The model under review builds one solid part; all positions refer to its coordinate system, in mm. Coordinates: 2 decimals unless noted, no trailing zeros. Write each loop counter-clockwise with the first axis right and the second up, starting at its lowest first coordinate (ties: lowest second). Pieces come first, ordered by that corner, then holes.
1) Mouldability with a two-part tool opening along Y and no side actions: class faces 1 (the cylindrical face through (1.57, 47.65, -37.69)), 2 (the flat face through (2, 51, 25.4)), 3 (the flat face through (1.57, 19.32, 12.88)) as released by +Y, released by -Y, zero draft, split by the parting line, or undercut.
2) Add section B-B, the plane z = -12.7. State the section outline as (x, y) points (3 decimals).
3) Add section A-A, the plane y = 50.8. State the section outline as (x, z) points (3 decimals), then the cut area to 3 significant figures.
4) For P1, Ø1, axis at x = 2, y = 28.5, coming from the +Z side, flat-tipped, find the tip position at first contact; note if it passes through.
5) Add section D-D, the plane y = 15. State the section outline as (x, z) points (3 decimals).
6) For line 1 (Z direction, x = 2.05, y = 50.8) (3 decimals); line 2 (Y direction, x = 1.2, z = -12.7) (3 decimals); line 3 (Z direction, x = 0.7, y = 48), list the stretches that pass through material, from the lowest coordinate up.
7) Add section C-C, the plane x = 2.1. State the section outline as (y, z) points (3 decimals).
Autodesk Inventor part; units mm, degrees
ref_plane "YZ Plane" through (0, 0, 0) normal (1, 0, 0) x (0, 1, 0)
ref_plane "XZ Plane" through (0, 0, 0) normal (0, 1, 0) x (-1, 0, 0)
ref_plane "XY Plane" through (0, 0, 0) normal (0, 0, 1) x (1, 0, 0)
sketch "Sketch1" plane through (0, 0, 0) normal (1, 0, 0) x (0, 1, 0)
  line L0 (0, 0) -> (0, -25.4)
  line L1 (0, -25.4) -> (38.1, -50.8)
  line L2 (38.1, -50.8) -> (63.5, -50.8)
  line L3 (63.5, -50.8) -> (63.5, 25.4)
  line L4 (63.5, 25.4) -> (38.1, 25.4)
  line L5 (38.1, 25.4) -> (0, 0)
  dimension "d0" = 76.2
  dimension "d2" = 25.4
  dimension "d3" = 25.4
  dimension "d4" = 25.4
  dimension "d5" = 63.5
  dimension "d6" = 25.4
extrude "Extrusion1" add sketch "Sketch1" along normal blind 3.175
sketch "Sketch2" plane through (3.175, 0, 0) normal (1, 0, 0) x (0, 0, -1)
  line L0 (0, 0) -> (25.4, 0)
  line L1 (50.8, 38.1) -> (50.8, 63.5)
  line L2 (50.8, 63.5) -> (-25.4, 63.5)
  line L3 (-25.4, 63.5) -> (-25.4, 38.1)
  point P0 (-12.7, 50.8)
  point P1 (38.1, 50.8)
  point P2 (12.7, 12.7)
  dimension "d9" = 12.7
  dimension "d10" = 12.7
  dimension "d11" = 12.7
  dimension "d12" = 12.7
  dimension "d13" = 12.7
  dimension "d14" = 12.7
hole "Hole1" at (3.175, 50.8, 12.7) at (3.175, 50.8, -38.1) at (3.175, 12.7, -12.7) direction (-1, 0, 0) diameter 6.35 end through all
properties part number "Mounting" material "Aluminum 6061"
Geometry results:
1. face 1: undercut
1. face 2: zero draft
1. face 3: released by -Y
2. outline: (0, 0) - (3.175, 0) - (3.175, 9.525) - (0, 9.525) - close; (0, 15.875) - (3.175, 15.875) - (3.175, 63.5) - (0, 63.5) - close
3. outline: (0, -50.8) - (3.175, -50.8) - (3.175, -41.275) - (0, -41.275) - close; (0, -34.925) - (3.175, -34.925) - (3.175, 9.525) - (0, 9.525) - close; (0, 15.875) - (3.175, 15.875) - (3.175, 25.4) - (0, 25.4) - close
3. area: 202 mm2
4. P1: stops at z = 19.33
5. outline: (0, -35.4) - (3.175, -35.4) - (3.175, -14.889) - (0, -14.889) - close; (0, -10.511) - (3.175, -10.511) - (3.175, 10) - (0, 10) - close
6. line 1: z = -50.8 to -41.275, -34.925 to 9.525, 15.875 to 25.4
6. line 2: y = 0 to 9.525, 15.875 to 63.5
6. line 3: z = -50.8 to -39.6, -36.6 to 11.2, 14.2 to 25.4
7. outline: (0, -25.4) - (38.1, -50.8) - (63.5, -50.8) - (63.5, 25.4) - (38.1, 25.4) - (0, 0) - close; hole circle Ø6.35 at (12.7, -12.7); hole circle Ø6.35 at (50.8, -38.1); hole circle Ø6.35 at (50.8, 12.7)
